The listing builds one solid part. Answer for the finished solid, in the listing's coordinates (mm). A direction names the side the tool comes from. Round coordinates to 2 decimals unless told otherwise and drop trailing zeros. Write each loop counter-clockwise with the first axis right and the second up, starting at its lowest first coordinate (ties: lowest second). Pieces come first, ordered by that corner, then holes. Notation, with made-up numbers: M 70.5,19 L 104.5,19 A30 ccw 104.5,46 Z; hole C -19.5,-10.75 d7. An arc over 180 degrees is marked long. Put each result on its own line as item: value. Start each with the question number.
```python
from build123d import *

# Parameters (mm, degrees)
ESQUISSE1_W        = 86.5
ESQUISSE1_H        = 60
ESQUISSE1_W_2      = 24.98
ESQUISSE1_H_2      = 5
BOSS_EXTRU_1_DEPTH = 6


with BuildPart() as part:
    # Esquisse1 → Boss.-Extru.1 (new body)
    with BuildSketch(Plane.XY):
        with Locations((16.736924874, 25.769230769)):
            Rectangle(ESQUISSE1_W, ESQUISSE1_H)
        with Locations((-7.013075126, -6.730769231)):
            Rectangle(ESQUISSE1_W_2, ESQUISSE1_H_2)
        with Locations((40.486924874, -6.730769231)):
            Rectangle(ESQUISSE1_W_2, ESQUISSE1_H_2)
    extrude(amount=BOSS_EXTRU_1_DEPTH)


solid = part.part
```
Item 1: Which of the six approach directions +Z, -Z, +X, -X, +Y, -Y give full straight-line access (tool end or side, diameter ignored) to faces 1 (the flat face through (52.977, -7, 3)), 2 (the flat face through (-19.503, -7, 3)), 3 (the flat face through (5.477, -7, 3))?
Item 2: Determine the mould class of faces 4 (the flat face through (59.987, 25, 3)), 5 (the flat face through (17, -4.231, 3)), 6 (the flat face through (16, 24, 6)) for opening direction X: released by +X, released by -X, zero draft, split by the parting line, or undercut.
Item 3: Section A-A (z = 3.65) is taken. Give the vertices of the cut face in (x, y).
Item 4: Flat-ended cylindrical pins translate along their axes: pin 1 (10 mm diameter, centred on x = 49, y = 34.5, fed in from -Z); pin 2 (3 mm diameter, centred on x = 22.5, z = 1.5, fed in from -Y); pin 3 (1.5 mm diameter, centred on y = -5.5, z = 3, fed in from -X); pin 4 (1.5 mm diameter, centred on y = -8, z = 1.5, fed in from +X). Find the tip coordinate at first contact, or state that the pin passes through.
Item 5: Consider line 1 along X through (y, z) = (-5.5, 0.9); line 2 along Y through (x, z) = (-20, 0.3). Determine where each line is inside the solid, lowest interval first. Write a range as [from, to].
Output values:
1. face 1: +Z, -Z, +X, -Y
1. face 2: +Z, -Z, -X, -Y
1. face 3: +Z, -Z, -Y
2. face 4: released by +X
2. face 5: undercut
2. face 6: zero draft
3. outline: M -26.51,-4.23 L -19.5,-4.23 L -19.5,-9.23 L 5.48,-9.23 L 5.48,-4.23 L 28,-4.23 L 28,-9.23 L 52.98,-9.23 L 52.98,-4.23 L 59.99,-4.23 L 59.99,55.77 L -26.51,55.77 Z
4. pin 1: stops at z = 0
4. pin 2: stops at y = -4.23
4. pin 3: stops at x = -19.5
4. pin 4: stops at x = 52.98
5. line 1: x = [-19.5, 5.48], [28, 52.98]
5. line 2: y = [-4.23, 55.77]
